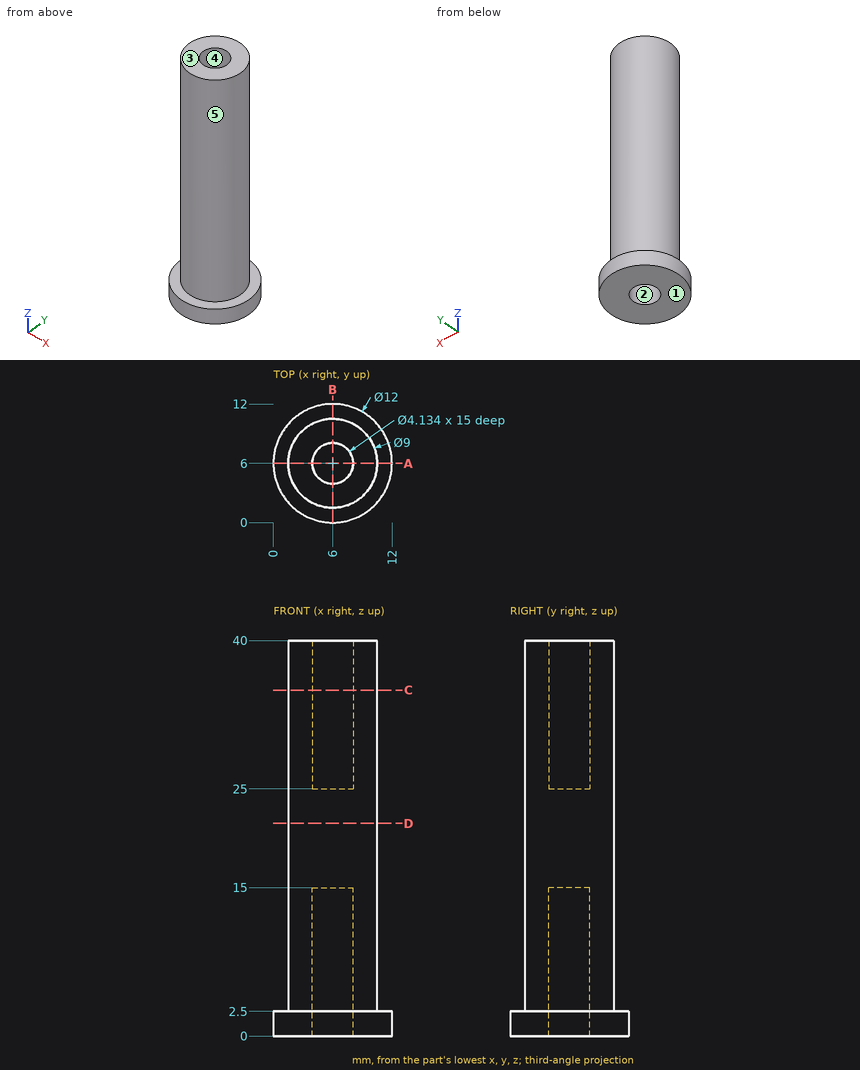
Print and shaded views of the part. All mm, measured from the part's lowest x, y and z. A direction names the side the tool comes from. Coordinates: 2 decimals unless noted, no trailing zeros. Order: outer loops, then holes, each group sorted by start corner. A loop starts at its lowest first (then second) coordinate and runs counter-clockwise, first axis right, second up. Notation, with made-up numbers: (-30, 33.25) - (-13, 33.25) arc R18 ccw to (-13, 44.25) - close; hole circle Ø8 at (8, 83.5). An arc over 180 degrees is marked (long way). Return JSON: item names as keys, results as strings. Group by question number.
Item 1: Cut at A-A (y = 6). List the corners of the cut face in (x, z).
Item 2: Drill centre lines: probe 1 along X at (y, z) = (6, 28.75); probe 2 along Y at (x, z) = (2, 20.5). Where is each one in solid material? Low to high. Write a range as from..to.
Item 3: Pull direction X, two halves, no side cores. Call the marked faces 3, 4 and 5: pulls with the +X half, pulls with the -X half, needs draft (parallel to the pull), parting line crosses it, or undercut.
Item 4: Which spindle directions (+Z, -Z, +X, -X, +Y, -Y) get a long thin tool onto all of the face, cutting with end or side? Do the marked faces 1 and 2. Say none if no direction does.
Item 5: Pin check, flat tips, straight feed: pin 1 (2.5 mm diameter, centred on x = 6, y = 6, fed in from +Z); pin 2 (4 mm diameter, centred on y = 5, z = 20.5, fed in from +X); pin 3 (1 mm diameter, centred on x = 8.5, z = 22.5, fed in from +Y). Stop position of each tip, or through.
Item 6: Cut at C-C (z = 35). List the corners of the cut face in (x, y).
Item 7: Cut at D-D (z = 21.5). List the corners of the cut face in (x, y), plus the area to 3 significant figures.
Check values:
{
 "1": {"outline": "(0, 0) - (3.93, 0) - (3.93, 15) - (8.07, 15) - (8.07, 0) - (12, 0) - (12, 2.5) - (10.5, 2.5) - (10.5, 40) - (8.07, 40) - (8.07, 25) - (3.93, 25) - (3.93, 40) - (1.5, 40) - (1.5, 2.5) - (0, 2.5) - close"},
 "2": {"probe 1": "x = 1.5..3.93, 8.07..10.5", "probe 2": "y = 3.94..8.06"},
 "3": {"face 3": "needs draft", "face 4": "undercut", "face 5": "parting line crosses it"},
 "4": {"face 1": "-Z, +X, -X, +Y, -Y", "face 2": "-Z"},
 "5": {"pin 1": "stops at z = 25", "pin 2": "stops at x = 10.5", "pin 3": "stops at y = 10.03"},
 "6": {"outline": "circle Ø9 at (6, 6); hole circle Ø4.13 at (6, 6)"},
 "7": {"outline": "circle Ø9 at (6, 6)", "area": "63.6 mm2"}
}
